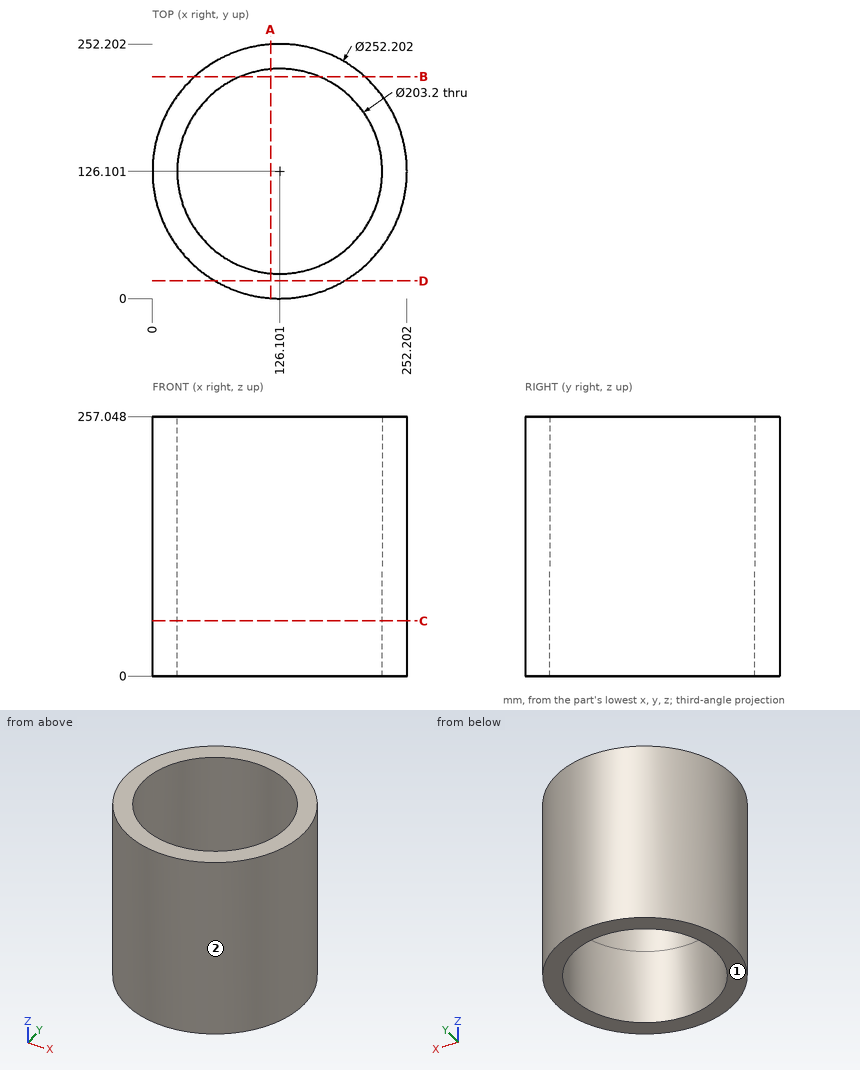
Source: three-view drawing plus pictorial views. Frame: mm from the lowest corner of the part. Round coordinates to 2 decimals unless told otherwise and drop trailing zeros. Order: outer loops, then holes, each group sorted by start corner. A loop starts at its lowest first (then second) coordinate and runs counter-clockwise, first axis right, second up. Notation, with made-up numbers: M 23.25,33 L 62.25,33 A28 ccw 62.25,61 Z; hole C -8,31 d6. An arc over 180 degrees is marked long. One line per item, written item: value.
(1) Line query: probe 1 along X at (y, z) = (128, 21.5) (1 decimal); probe 2 along Y at (x, z) = (152.5, 48.5) (1 decimal); probe 3 along Y at (x, z) = (66, 115.5) (1 decimal). Output: solid intervals per line, ascending. Write a range as [from, to].
Result sheet:
probe 1: [0, 24.5], [227.7, 252.2]
probe 2: [2.8, 28], [224.2, 249.4]
probe 3: [15.2, 44.2], [208, 237]
(2) Cut plane B-B (y = 220). Return the cut outline in (x, z), and give its area (3 significant figures).
Result sheet:
outline: M 41.93,0 L 87.3,0 L 87.3,257.05 L 41.93,257.05 Z; M 164.9,0 L 210.27,0 L 210.27,257.05 L 164.9,257.05 Z
area: 23,300 mm2
(3) Cut plane C-C (z = 54.5). Return the cut outline in (x, y).
Result sheet:
outline: C 126.1,126.1 d252.2; hole C 126.1,126.1 d203.2
(4) Cut plane A-A (x = 117). Return the cut outline in (y, z).
Result sheet:
outline: M 0.33,0 L 24.91,0 L 24.91,257.05 L 0.33,257.05 Z; M 227.29,0 L 251.87,0 L 251.87,257.05 L 227.29,257.05 Z
(5) Cut plane D-D (y = 17.5). Return the cut outline in (x, z).
Result sheet:
outline: M 62.01,0 L 190.19,0 L 190.19,257.05 L 62.01,257.05 Z
(6) Pin query (flat end, axial travel): P1, Ø10, axis at y = 168, z = 169.5, coming from the -X side; P2, Ø1, axis at y = 68.5, z = 65.5, coming from the -X side; P3, Ø5, axis at x = 218, z = 73.5, coming from the -Y side (1 decimal). Return the tip coordinate at first contact, or that it passes through.
Result sheet:
P1: x = 5.52
P2: x = 13.67
P3: y = 37.2
(7) Pull-direction query (X, two-part tool) for the marked faces 1 and 2; classes: pulls with the +X half, pulls with the -X half, needs draft (parallel to the pull), parting line crosses it, or undercut.
Result sheet:
face 1: needs draft
face 2: parting line crosses it
